Autodesk Inventor part; units mm, degrees
ref_plane "Work Plane1" through (-10.2594, 70.1311, 132.15) normal (0.9396926, -0.3420201, 0) x (0, 0, -1)
ref_plane "Work Plane2" through (72.1517, 40.136, 4) normal (0, 0, -1) x (-0.9396926, 0.3420201, 0)
ref_plane "YZ Plane" through (0, 0, 0) normal (1, 0, 0) x (0, 1, 0)
sketch "Sketch1" plane through (0, 0, 0) normal (0, 1, 0) x (-1, 0, 0)
  line L0 (100, 155) -> (-100, 155)
  line L1 (-100, 155) -> (-100, -155)
  line L2 (-100, -155) -> (100, -155)
  line L3 (100, -155) -> (100, 155)
  point P0 (0, 0)
  point P1 (100, 0)
  point P2 (0, -155)
  dimension "d0" = 310
  dimension "d1" = 200
sketch "Sketch2" plane through (0, 0, 0) normal (0, 0, 1) x (1, 0, 0)
  line L0 (-100, 0) -> (100, 0)
  line L1 (100, 0) -> (100, 30)
  line L2 (100, 30) -> (-100, 102.794)
  line L3 (-100, 0) -> (-100, 102.794)
  line L4 (-96, 97.0815) -> (96, 27.1992)
  line L5 (96, 27.1992) -> (96, 0)
  line L6 (-96, 0) -> (-96, 97.0815)
  point P0 (0, 0)
  point P1 (0, 0)
  dimension "d2" = 200
  dimension "d3" = 30
  dimension "d4" = 110
  dimension "d5" = 4
  dimension "d6" = 110
  dimension "d7" = 4
  dimension "d8" = 27.1992
extrude "Extrusion1" add sketch "Sketch2" along normal mid plane 310
extrude "Extrusion2" cut sketch "Sketch2" along normal mid plane 302 contours L6 L4 L5 L0
sketch "Sketch3" plane through (-100, 102.794, 155) normal (0.3420201, 0.9396926, 0) x (0.9396926, -0.3420201, 0)
  line L0 (27.85, 15) -> (183.2, 15)
  line L1 (191.05, 22.85) -> (191.05, 263.3)
  line L2 (183.2, 271.15) -> (27.85, 271.15)
  line L3 (20, 263.3) -> (20, 22.85)
  line L4 (0, 310) -> (0, 0)
  line L5 (212.8356, 0) -> (0, 0)
  arc A0 (20, 22.85) -> (27.85, 15) centre (27.85, 22.85) ccw
  arc A1 (27.85, 271.15) -> (20, 263.3) centre (27.85, 263.3) ccw
  arc A2 (191.05, 263.3) -> (183.2, 271.15) centre (183.2, 263.3) ccw
  arc A3 (183.2, 15) -> (191.05, 22.85) centre (183.2, 22.85) ccw
  point P0 (129.1269, 155)
  point P1 (191.05, 271.15)
  point P2 (191.05, 15)
  point P3 (20, 271.15)
  dimension "d13" = 171.05
  dimension "d14" = 256.15
  dimension "d15" = 20
  dimension "d16" = 15
  dimension "d17" = 7.85
  dimension "d18" = 7.85
extrude "Extrusion3" cut sketch "Sketch3" against normal up to next
fillet "Fillet1" radius 5 4 edges at (0, 66.397, 155) (0, 66.397, -155) (-100, 102.794, 0) (100, 30, 0)
ref_plane "Work Plane1" through (-10.2594, 70.1311, 132.15) normal (0.9396926, -0.3420201, 0) x (0, 0, -1)
sketch "Sketch4" plane through (-10.2594, 70.1311, 132.15) normal (0.9396926, -0.3420201, 0) x (0, 0, -1)
  point P0 (132.15, -62.3928)
ref_plane "Work Plane2" through (72.1517, 40.136, 4) normal (0, 0, -1) x (-0.9396926, 0.3420201, 0)
sketch "Sketch5" plane through (72.1517, 40.136, 4) normal (0, 0, -1) x (-0.9396926, 0.3420201, 0)
  point P0 (54.0731, -62.3928)
fillet "Fillet2" radius 3 1 edges at (-96, 97.0815, 0)
properties part number "Screen_Support"
Source: CAD feature listing. Evaluate the final solid. Frame: model axes, mm. A direction names the side the tool comes from. Give positions to 0.01 mm unless a question says otherwise; leave off trailing zeros. Write each loop counter-clockwise with the first axis right and the second up, starting at its lowest first coordinate (ties: lowest second). Pieces come first, ordered by that corner, then holes. Notation, with made-up numbers: (50.25, 69) - (61.25, 69) arc R22 cw to (61.25, 87) - close; hole circle Ø11 at (89, 0). An arc over 180 degrees is marked (long way). Write item = value, one per line. Start each with the question number.
Q1. Material intervals for probe 1 along Z at (x, y) = (-73, 75); probe 2 along X at (y, z) = (25, 16.5); probe 3 along X at (y, z) = (65, -101.5), sorted ascending.
Q2. Reachability of faces 5 (the cylindrical face through (76.64, 36.41, 137.76)), 6 (the cylindrical face through (-79.662, 93.293, -113.911)), 7 (the flat face through (-24, 39, 155)), 8 (the flat face through (96, 14, -2)), 9 (the cylindrical face through (-97.92, 99.71, -2.17)) from +Z, -Z, +X, -X, +Y, -Y: full face, straight path, thin tool, end or side. Return the list, or none.
Q3. Pin query (flat end, axial travel): pin 1 Ø10 at (y, z) = (61, 44.5) entering from +X. Return the tip coordinate at first contact, or that it passes through.
Q4. Cut plane A-A, the plane z = -89. Return loops of the section in (x, y).
Q5. Cut plane B-B, the plane y = 12.5. Return loops of the section in (x, z), then the cut area to 3 significant figures.
Q6. Draft query along X for faces 1 (the flat face through (-97, 0, -1)), 2 (the flat face through (-23, 38, 151)), 3 (the flat face through (100, 13, -2)), 4 (the flat face through (-96, 46, -2)). Return one class per face: +X half, -X half, draft (parallel to the pull), parting line (faces both ways), or undercut.
Q7. Cut plane C-C, the plane z = 136.5. Return loops of the section in (x, y), then the cut area to 3 significant figures.
Computed values:
q1.probe_1 = -155 to -151, 151 to 155
q1.probe_2 = -100 to -96, 96 to 100
q1.probe_3 = -100 to -96
q2.face_5 = +Y
q2.face_6 = +X, -Y
q2.face_7 = +Z, +X, -X, +Y, -Y
q2.face_8 = -Y
q2.face_9 = +Z, -Z, +Y
q3.pin_1 = -96
q4.outline = (-100, 0) - (-96, 0) - (-96, 92.8) arc R3 cw to (-91.97, 95.62) - (-82.57, 92.19) - (-81.21, 95.95) - (-93.29, 100.35) arc R5 ccw to (-100, 95.65) - close; (78.16, 33.69) - (96, 27.2) - (96, 0) - (100, 0) - (100, 26.5) arc R5 ccw to (96.71, 31.2) - (79.53, 37.45) - close
q5.outline = (-100, -155) - (100, -155) - (100, 155) - (-100, 155) - close; hole (-96, -151) - (96, -151) - (96, 151) - (-96, 151) - close
q5.area = 4,020 mm²
q6.face_1 = draft
q6.face_2 = undercut
q6.face_3 = +X half
q6.face_4 = undercut
q7.outline = (-100, 0) - (-96, 0) - (-96, 92.8) arc R3 cw to (-91.97, 95.62) - (-81.34, 91.74) - (-79.97, 95.5) - (-93.29, 100.35) arc R5 ccw to (-100, 95.65) - close; (76.92, 34.14) - (96, 27.2) - (96, 0) - (100, 0) - (100, 26.5) arc R5 ccw to (96.71, 31.2) - (78.29, 37.9) - close
q7.area = 665 mm²
